Autodesk Inventor part; units mm, degrees
ref_plane "YZ Plane" through (0, 0, 0) normal (1, 0, 0) x (0, 1, 0)
ref_plane "XZ Plane" through (0, 0, 0) normal (0, 1, 0) x (-1, 0, 0)
ref_plane "XY Plane" through (0, 0, 0) normal (0, 0, 1) x (1, 0, 0)
sketch "Sketch1" plane through (0, 0, 0) normal (0, 1, 0) x (-1, 0, 0)
  circle A0 centre (0, 0) radius 12.7
  circle A1 centre (0, 0) radius 3.302
  dimension "d0" = 25.4
  dimension "d1" = 6.604
extrude "Extrusion1" add sketch "Sketch1" along normal blind 6.35
sketch "Sketch2" plane through (0, 6.35, 0) normal (0, 1, 0) x (1, 0, 0)
  line L0 (0, 0) -> (0, -5.08)
  line L1 (0, -5.08) -> (0, 0)
  line L2 (0, 0) -> (0, 5.08)
  circle A0 centre (0, -5.08) radius 1.1049
  circle A1 centre (0, 5.08) radius 1.1049
  dimension "d4" = 5.08
  dimension "d5" = 5.08
  dimension "d6" = 2.2098
  dimension "d7" = 2.2098
extrude "Extrusion2" cut sketch "Sketch2" against normal blind 4.445
sketch "Sketch3" plane through (0, 0, 0) normal (0, -1, 0) x (1, 0, 0)
  line L0 (0, 0) -> (0, 5.08)
  line L1 (0, 5.08) -> (0, -5.08)
  circle A0 centre (0, 5.08) radius 1.1049
  circle A1 centre (0, -5.08) radius 1.1049
  dimension "d10" = 5.08
  dimension "d11" = 10.16
  dimension "d14" = 2.2098
  dimension "d15" = 2.2098
extrude "Extrusion3" cut sketch "Sketch3" against normal blind 1.905
properties part number "PolarisPost_HeightAdjustment_0p25in_smallholesfrom0p79to0p81"
Here's how the part is built. I have some questions about the finished solid (model axes, mm). Give positions to 0.01 mm unless a question says otherwise; leave off trailing zeros. Order: outer loops, then holes, each group sorted by start corner. A loop starts at its lowest first (then second) coordinate and runs counter-clockwise, first axis right, second up. Notation, with made-up numbers: (27.25, 16) -> (74.25, 16) arc R14 ccw to (74.25, 42) -> close; hole circle Ø6 at (-35, -30). An arc over 180 degrees is marked (long way). Use CSV: the item, a comma, the result in double quotes. Start each with the question number.
Item 1: Suppose I cut it at D-D (y = 2). List the corners of the cut face in (x, z) for me.
Item 2: Thinking about a two-plate mould opening in Z: for faces 1 (the flat face through (-3, 0, -3)), 2 (the cylindrical face through (2.75, 3.13, 12.4)), 3 (the cylindrical face through (-3.05, 3.13, 1.26)), which applies, pulls with the +Z half, pulls with the -Z half, needs draft (parallel to the pull), parting line crosses it, or undercut?
Item 3: Suppose I cut it at A-A (z = 0). List the corners of the cut face in (x, y) for me, and give its area (3 significant figures).
Item 4: Suppose I cut it at B-B (x = 0). List the corners of the cut face in (y, z) for me.
Item 5: If I drill on probe 1 along Z at (x, y) = (0, 2.5); probe 2 along Z at (x, y) = (0.75, 5); probe 3 along X at (y, z) = (3.5, 5.08), over which ranges is the centre line in solid material (lowest first)? Write a range as [from, to].
Item 6: I'm going to push flat-ended pins straight in: P1, Ø2, axis at x = 7.5, y = 1, coming from the +Z side; P2, Ø8, axis at x = 6.5, z = -3.5, coming from the -Y side; P3, Ø2, axis at y = 2.5, z = 5.5, coming from the +X side; P4, Ø1, axis at x = 5.5, y = 5.5, coming from the +Z side. Where does each tip first touch, or does it pass through?
Item 7: Suppose I cut it at C-C (x = 3). List the corners of the cut face in (y, z) for me.
Answer block:
1,outline,"circle Ø25.4 at (0, 0); hole circle Ø6.6 at (0, 0); hole circle Ø2.21 at (0, -5.08); hole circle Ø2.21 at (0, 5.08)"
2,face 1,"needs draft"
2,face 2,"parting line crosses it"
2,face 3,"undercut"
3,outline,"(-12.7, 0) -> (-3.3, 0) -> (-3.3, 6.35) -> (-12.7, 6.35) -> close; (3.3, 0) -> (12.7, 0) -> (12.7, 6.35) -> (3.3, 6.35) -> close"
3,area,"119 mm^2"
4,outline,"(0, -12.7) -> (6.35, -12.7) -> (6.35, -6.18) -> (0, -6.18) -> close; (0, -3.98) -> (6.35, -3.98) -> (6.35, -3.3) -> (0, -3.3) -> close; (0, 3.3) -> (6.35, 3.3) -> (6.35, 3.98) -> (0, 3.98) -> close; (0, 6.18) -> (6.35, 6.18) -> (6.35, 12.7) -> (0, 12.7) -> close"
5,probe 1,"z = [-12.7, -6.18], [-3.98, -3.3], [3.3, 3.98], [6.18, 12.7]"
5,probe 2,"z = [-12.68, -5.89], [-4.27, -3.22], [3.22, 4.27], [5.89, 12.68]"
5,probe 3,"x = [-11.64, -1.1], [1.1, 11.64]"
6,P1,"stops at z = 10.91"
6,P2,"stops at y = 0"
6,P3,"stops at x = 11.88"
6,P4,"stops at z = 11.67"
7,outline,"(0, -12.34) -> (6.35, -12.34) -> (6.35, -1.38) -> (0, -1.38) -> close; (0, 1.38) -> (6.35, 1.38) -> (6.35, 12.34) -> (0, 12.34) -> close"
